from build123d import *
from build123d.topology import SkipClean

# Parameters (mm, degrees)
SKETCH2_R               = 120
BOSS_EXTRUDE2_DEPTH     = 85
CUT_EXTRUDE1_START      = -82
CUT_EXTRUDE1_DEPTH      = 82
CUT_EXTRUDE5_DEPTH      = 2
CUT_EXTRUDE5_DEPTH_BACK = 2
SKETCH8_R               = 75
SKETCH9_R               = 32
CUT_EXTRUDE6_DEPTH      = 5
BOSS_EXTRUDE4_START     = 40
SKETCH12_R              = 32
BOSS_EXTRUDE4_DEPTH     = 40


with BuildPart() as part:
    # Sketch2 → Boss-Extrude2 (new body)
    with BuildSketch(Plane.XY):
        Circle(SKETCH2_R)
    extrude(amount=BOSS_EXTRUDE2_DEPTH)

    # Sketch3 → Cut-Extrude1 (cut)
    with BuildSketch(Plane.XY.offset(85).offset(CUT_EXTRUDE1_START)):
        with BuildLine():
            Line((-108.885260711, -40), (-113.13708499, -40))
            ThreePointArc((-113.13708499, -40), (0, -120), (113.13708499, -40))
            Line((113.13708499, -40), (108.885260711, -40))
            ThreePointArc((108.885260711, -40), (0, 116), (-108.885260711, -40))
        make_face()
    extrude(amount=CUT_EXTRUDE1_DEPTH, mode=Mode.SUBTRACT)

    # Sketch8 → Cut-Extrude5 (cut, two sides: drawn at the far end of the back side and taken through both)
    with BuildSketch(Plane.XY.offset(3).offset(-CUT_EXTRUDE5_DEPTH_BACK)):
        Circle(SKETCH8_R)
    extrude(amount=CUT_EXTRUDE5_DEPTH + CUT_EXTRUDE5_DEPTH_BACK, mode=Mode.SUBTRACT)

    # Sketch9 → Cut-Extrude6 (cut)
    with BuildSketch(Plane.XY.offset(1)):
        Circle(SKETCH9_R)
    extrude(amount=-CUT_EXTRUDE6_DEPTH, mode=Mode.SUBTRACT)

    # Sketch12 → Boss-Extrude4 (add)
    # profile 1 of 2: a face of its own
    with SkipClean():  # the faces are left unmerged after this step: merging them gives an invalid solid
        with BuildSketch(Plane(origin=(0, 0, 0), x_dir=(-1, 0, 0), z_dir=(0, 0, -1)).offset(BOSS_EXTRUDE4_START)):
            with BuildLine():
                ThreePointArc((120, 0), (0, 120), (-120, 0))
                Line((-120, 0), (-118.831087629, -16.70845932))
                ThreePointArc((-118.831087629, -16.70845932), (-3.111785776, -119.959646504), (117.805011812, -22.84686394))
                Line((117.805011812, -22.84686394), (120, 0))
            make_face()
            with Locations(Location((0, 0, 0), (0, 0, 180))):
                Circle(SKETCH12_R, mode=Mode.SUBTRACT)
        # profile 2 of 2: a face of its own
        with BuildSketch(Plane(origin=(0, 0, 0), x_dir=(-1, 0, 0), z_dir=(0, 0, -1)).offset(BOSS_EXTRUDE4_START)):
            with BuildLine():
                ThreePointArc((117.805011812, -22.84686394), (-3.111785776, -119.959646504), (-118.831087629, -16.70845932))
                Line((-118.831087629, -16.70845932), (-99.063378042, -299.268538041))
                ThreePointArc((-99.063378042, -299.268538041), (-3.575656086, -388.008129656), (91.309922092, -298.624981255))
                Line((91.309922092, -298.624981255), (117.805011812, -22.84686394))
            make_face()
        extrude(amount=-BOSS_EXTRUDE4_DEPTH)


solid = part.part
Could you check a few things on this model? Use its own coordinates, in mm. A direction names the side the tool comes from. Round coordinates to 2 decimals unless told otherwise and drop trailing zeros. Write each loop counter-clockwise with the first axis right and the second up, starting at its lowest first coordinate (ties: lowest second). Pieces come first, ordered by that corner, then holes. Notation, with made-up numbers: (73.25, -20.75) -> (88.25, -20.75) arc R22 cw to (88.25, 1.25) -> close; hole circle Ø2 at (61.25, -8). An arc over 180 degrees is marked (long way). Use a Markdown table: item, result.
1. If we section it at B-B (y = 6.5): List the corners of the cut face in (x, z) for me.
Answer key:
| item | result |
|---|---|
| outline | (-119.82, -40) -> (-31.33, -40) -> (-31.33, 1) -> (-74.72, 1) -> (-74.72, 3) -> (-115.82, 3) -> (-115.82, 85) -> (-119.82, 85) -> close; (31.33, -40) -> (119.82, -40) -> (119.82, 85) -> (115.82, 85) -> (115.82, 3) -> (74.72, 3) -> (74.72, 1) -> (31.33, 1) -> close |
2. Which directions (+Z, -Z, +X, -X, +Y, -Y) give clear straight access to the entire face, cutting with the end or side of a thin tool? Please do faces 1 (the face through (32.3, 1, 1)), 2 (the face through (2, -130, -40)).
Answer key:
| item | result |
|---|---|
| face 1 | +Z |
| face 2 | -Z, +X, -X, +Y, -Y |
3. Please list where these lines run through material, in increasing order: probe 1 along X at (y, z) = (0, 44); probe 2 along Y at (x, z) = (0, -30.5); probe 3 along Y at (x, z) = (0, 2).
Answer key:
| item | result |
|---|---|
| probe 1 | x = -120 to -116, 116 to 120 |
| probe 2 | y = -387.93 to -32, 32 to 120 |
| probe 3 | y = -120 to -75, 75 to 120 |
4. For pin 1 Ø2 at (x, z) = (-111, 37.5) entering from -Y; pin 2 Ø4 at (y, z) = (24, 48.5) entering from +X; pin 3 Ø4 at (x, y) = (-75, -80.5) entering from +Z, each with a flat end and sliding along its axis, tell me the tip position at first contact or that it passes through.
Answer key:
| item | result |
|---|---|
| pin 1 | stops at y = -40 |
| pin 2 | stops at x = 117.97 |
| pin 3 | stops at z = 3 |
5. If we section it at D-D (y = -93.5): List the corners of the cut face in (x, z) for me, then the cut area to 3 significant figures.
Answer key:
| item | result |
|---|---|
| outline | (-111.02, -40) -> (113.46, -40) -> (113.46, 0) -> (75.22, 0) -> (75.22, 3) -> (-75.22, 3) -> (-75.22, 0) -> (-111.02, 0) -> close |
| area | 9,430 mm^2 |
6. We'd pull the mould along Y, two halves only. Please class faces 3 (the face through (5.585, -387.994, -20.28)), 4 (the face through (-36, 111, 85)), 5 (the face through (3.12, 115.96, 43.43)), 6 (the face through (-6.94, 31.24, -19.79)): +Y half, -Y half, draft (parallel to the pull), parting line (faces both ways), or undercut.
Answer key:
| item | result |
|---|---|
| face 3 | -Y half |
| face 4 | draft |
| face 5 | undercut |
| face 6 | undercut |
7. If we section it at A-A (z = -26): List the corners of the cut face in (x, y) for me, then the cut area to 3 significant figures.
Answer key:
| item | result |
|---|---|
| outline | (-120, 0) -> (-91.31, -298.62) arc R95.4 ccw to (99.06, -299.27) -> (120, 0) arc R120 ccw to start; hole circle Ø64 at (0, 0) |
| area | 96,800 mm^2 |
8. If we section it at C-C (x = 0): List the corners of the cut face in (y, z) for me, then the cut area to 3 significant figures.
Answer key:
| item | result |
|---|---|
| outline | (-387.93, -40) -> (-32, -40) -> (-32, 1) -> (-75, 1) -> (-75, 3) -> (-120, 3) -> (-120, 0) -> (-387.93, 0) -> close; (32, -40) -> (120, -40) -> (120, 85) -> (116, 85) -> (116, 3) -> (75, 3) -> (75, 1) -> (32, 1) -> close |
| area | 18,400 mm^2 |
